Geometry: final body of the model. Coordinates: model frame, mm. Give positions to 0.01 mm unless a question says otherwise; leave off trailing zeros. Write each loop counter-clockwise with the first axis right and the second up, starting at its lowest first coordinate (ties: lowest second). Pieces come first, ordered by that corner, then holes.
Q1. Section B-B (x = -4.25). Return the cut outline in (y, z).
Q2. Line query: line 1 (Y direction, x = 0, z = 76.25); line 2 (X direction, y = 0.5, z = -57.5); line 3 (X direction, y = -3.75, z = -69). Output: solid intervals per line, ascending.
Q3. Section A-A (z = -25). Return the cut outline in (x, y), plus the area to 3 significant figures.
Q4. Pin query (flat end, axial travel): pin 1 Ø1.5 at (x, y) = (0, 0) entering from +Z; pin 2 Ø2 at (y, z) = (3, -53) entering from +X; pin 3 Ø2 at (x, z) = (-1, -41) entering from -Y; pin 4 Ø2 at (x, y) = (0, 0) entering from +Z. Return the tip coordinate at first contact, or that it passes through.
Q5. Section C-C (y = -2.75). Return the cut outline in (x, z), plus the area to 3 significant figures.
from build123d import *

# Parameters (mm, degrees)
SKETCH2_R           = 6
BOSS_EXTRUDE1_DEPTH = 83.5


with BuildPart() as part:
    # Sketch2 → Boss-Extrude1 (new body, symmetric)
    with BuildSketch(Plane.XY):
        Circle(SKETCH2_R)
    extrude(amount=BOSS_EXTRUDE1_DEPTH, both=True)

    # Sketch4 → Tap Drill for M3x0.5 Tap1 (revolve, cut)
    with BuildSketch(Plane(origin=(0, 0, 83.5), x_dir=(0, -1, 0), z_dir=(1, 0, 0))):
        Polygon((0, 0), (0, 10.751075774), (1.25, 10), (1.25, 0), align=None)
    tap_drill_for_m3x0_5_tap1 = revolve(axis=Axis((0, 0, 89.85), (0, 0, -1)), mode=Mode.SUBTRACT)

    # Mirror1: Tap Drill for M3x0.5 Tap1 across plane
    add(tap_drill_for_m3x0_5_tap1.mirror(Plane.XY), mode=Mode.SUBTRACT)


solid = part.part
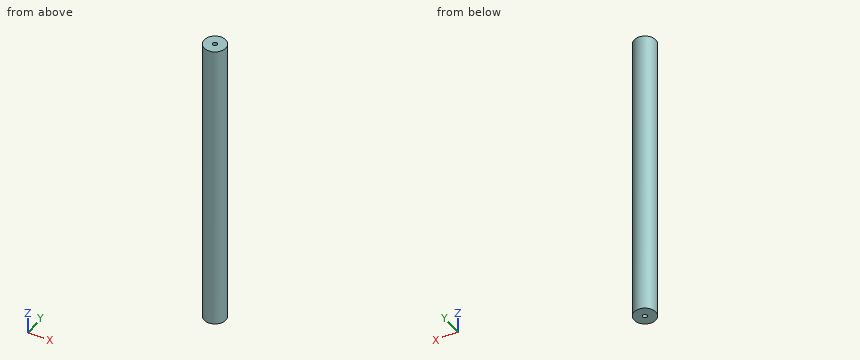
Computed:
1. outline: (-4.24, -83.5) - (4.24, -83.5) - (4.24, 83.5) - (-4.24, 83.5) - close
2. line 1: y = -6 to -1.25, 1.25 to 6
2. line 2: x = -5.98 to 5.98
2. line 3: x = -4.68 to 4.68
3. outline: circle Ø12 at (0, 0)
3. area: 113 mm2
4. pin 1: stops at z = 73.2
4. pin 2: stops at x = 5.66
4. pin 3: stops at y = -6
4. pin 4: stops at z = 73.35
5. outline: (-5.33, -83.5) - (5.33, -83.5) - (5.33, 83.5) - (-5.33, 83.5) - close
5. area: 1,780 mm2
